```python
from build123d import *

# Parameters (mm, degrees)
COQUE1_T           = -1
ESQUISSE3_R        = 2.5
ESQUISSE3_R_2      = 1.5
BOSS_EXTRU_1_DEPTH = 3.2


with BuildPart() as part:
    # Esquisse2 → Lissage1 section 0
    with BuildSketch(Plane.XY.offset(5)):
        with BuildLine():
            Line((3.5, 3.5), (-3.5, 3.5))
            Line((-3.5, 3.5), (-3.5, -3.5))
            Line((-3.5, -3.5), (3.5, -3.5))
            Line((3.5, -3.5), (3.5, 3.5))
        make_face()
    # Esquisse1 → Lissage1 section 1
    with BuildSketch(Plane.XY):
        with BuildLine():
            Line((-3, 3), (3, 3))
            Line((3, 3), (3, -3))
            Line((3, -3), (-3, -3))
            Line((-3, -3), (-3, 3))
        make_face()
    loft()

    # Coque1
    coque1_openings = [part.faces().sort_by_distance(p)[0] for p in [
        (0, 0, 5),
    ]]
    offset(amount=COQUE1_T, openings=coque1_openings, kind=Kind.INTERSECTION)

    # Esquisse3 → Boss.-Extru.1 (add)
    with BuildSketch(Plane.XY.offset(1)):
        Circle(ESQUISSE3_R)
        Circle(ESQUISSE3_R_2, mode=Mode.SUBTRACT)
    extrude(amount=BOSS_EXTRU_1_DEPTH)


solid = part.part
```
Design review of the part built by this model. Coordinates are the model's own, in mm. A direction names the side the tool comes from. Round coordinates to 2 decimals unless told otherwise and drop trailing zeros.
Item 1: For faces 1 (the flat face through (0, 0, 0)), 2 (the flat face through (-2, 0, 4.2)), list the 3-axis set-ups (+Z, -Z, +X, -X, +Y, -Y) from which the entire face can be reached by the end or side of a thin tool; tool diameter is ignored.
Item 2: The part is to be moulded in two halves that separate along Y. For faces 3 (the cylindrical face through (1.781, 1.755, 2.933)), 4 (the flat face through (3, 0, 5)), 5 (the flat face through (0, 0, 1)), say which applies: +Y half, -Y half, draft (parallel to the pull), parting line (faces both ways), or undercut.
Item 3: Clearance check with flat-ended pins moving along their axes: pin 1 Ø1.5 at (x, z) = (2, 2.5) entering from -Y (3 decimals); pin 2 Ø1 at (y, z) = (-3, 0.5) entering from +X; pin 3 Ø2.5 at (x, y) = (0, 0) entering from +Z. State where each tip first meets the part, or that it passes through.
Item 4: For probe 1 along Y at (x, z) = (2.25, 3.25) (3 decimals); probe 2 along Y at (x, z) = (0, 3.45) (3 decimals); probe 3 along Z at (x, y) = (-1.5, 1.25), list the stretches that pass through material, from the lowest coordinate up.
Item 5: We need section A-A on z = 3. State how many separate pieces and enclosed holes the cut face has, and give its area (3 significant figures).
Returned:
1. face 1: -Z, +X, -X, +Y, -Y
1. face 2: +Z
2. face 3: undercut
2. face 4: draft
2. face 5: undercut
3. pin 1: stops at y = -3.325
3. pin 2: stops at x = 3.1
3. pin 3: stops at z = 1
4. probe 1: y = -3.325 to -2.32, -1.09 to 1.09, 2.32 to 3.325
4. probe 2: y = -3.345 to -1.5, 1.5 to 3.345
4. probe 3: z = 0 to 4.2
5. separate pieces: 1
5. enclosed holes: 5
5. area: 34.0 mm2
